Could you check a few things on this model? Use its own coordinates, in mm. Give positions to 0.01 mm unless a question says otherwise; leave off trailing zeros. Order: outer loops, then holes, each group sorted by start corner. A loop starts at its lowest first (then second) coordinate and runs counter-clockwise, first axis right, second up. Notation, with made-up numbers: M 8.5,74 L 50.5,74 A6 ccw 50.5,79 Z; hole C 43.5,64.5 d7. An arc over 180 degrees is marked long. Use a Markdown table: item, result. Add a question column.
Item 1: Suppose I cut it at B-B on z = 164. Write out the boundary of the cut face in (x, y) (3 decimals), plus the area to 3 significant figures.
Item 2: I'm going to push flat-ended pins straight in: pin 1 Ø3 at (x, z) = (1, -208) entering from +Y; pin 2 Ø5.5 at (x, z) = (0, -30) entering from +Y; pin 3 Ø0.6 at (y, z) = (8.5, 53) entering from +X. Where does each tip first touch, or does it pass through?
Item 3: Suppose I cut it at A-A on y = 3.5. Count the separate pieces of the cut face and the enclosed holes in it, plus the area to 3 significant figures.
Item 4: If I drill on L1, parallel to X at y = 1.35, z = 30; L2, parallel to X at y = 7, z = -150; L3, parallel to Y at x = -8.5, z = 46, over which ranges is the centre line in solid material (lowest first)? Write a range as from..to.
from build123d import *

# Parameters (mm, degrees)
BOSS_EXTRUDE1_DEPTH      = 230
BOSS_EXTRUDE1_DEPTH_BACK = 230


with BuildPart() as part:
    # Sketch1 → Boss-Extrude1 (new, two sides: drawn at the far end of the back side and taken through both)
    with BuildSketch(Plane.XY.offset(-BOSS_EXTRUDE1_DEPTH_BACK)):
        with BuildLine():
            Line((-10, 6.77615), (-10, 0.5))
            Line((-10, 0.5), (-9.5, 0))
            Line((-9.5, 0), (9.5, 0))
            Line((9.5, 0), (10, 0.5))
            Line((10, 0.5), (10, 6.77615))
            Line((10, 6.77615), (9.440021531, 7.099443113))
            ThreePointArc((9.440021531, 7.099443113), (9.015681976, 7.442706235), (8.71772889, 7.9))
            Line((8.71772889, 7.9), (7.5, 7.9))
            Line((7.5, 7.9), (7.5, 9.1))
            Line((7.5, 9.1), (8.71772889, 9.1))
            ThreePointArc((8.71772889, 9.1), (9.015681976, 9.557293765), (9.440021531, 9.900556887))
            Line((9.440021531, 9.900556887), (10, 10.22385))
            Line((10, 10.22385), (10, 10.7))
            Line((10, 10.7), (9.7, 11))
            Line((9.7, 11), (-9.7, 11))
            Line((-9.7, 11), (-10, 10.7))
            Line((-10, 10.7), (-10, 10.22385))
            Line((-10, 10.22385), (-9.440021531, 9.900556887))
            ThreePointArc((-9.440021531, 9.900556887), (-9.015681976, 9.557293765), (-8.71772889, 9.1))
            Line((-8.71772889, 9.1), (-7.5, 9.1))
            Line((-7.5, 9.1), (-7.5, 7.9))
            Line((-7.5, 7.9), (-8.71772889, 7.9))
            ThreePointArc((-8.71772889, 7.9), (-9.015681976, 7.442706235), (-9.440021531, 7.099443113))
            Line((-9.440021531, 7.099443113), (-10, 6.77615))
        make_face()
    extrude(amount=BOSS_EXTRUDE1_DEPTH + BOSS_EXTRUDE1_DEPTH_BACK)

    # Sketch2 → Cut-Revolve1 (revolve, cut)
    with BuildSketch(Plane(origin=(0, 0, 0), x_dir=(0, 0, -1), z_dir=(1, 0, 0)), mode=Mode.PRIVATE) as cut_revolve1_sk:
        Polygon((210, 11), (214.75, 11), (214.75, 5.5), (213, 5.5), (213, 0), (210, 0), align=None)
    revolve(cut_revolve1_sk.sketch.rotate(Axis((0, 0, -210), (0, 1, 0)), 180), axis=Axis((0, 0, -210), (0, 1, 0)), mode=Mode.SUBTRACT)

    # Sketch3 → Cut-Revolve2 (revolve, cut)
    with BuildSketch(Plane(origin=(0, 0, 0), x_dir=(0, 0, -1), z_dir=(1, 0, 0)), mode=Mode.PRIVATE) as cut_revolve2_sk:
        Polygon((150, 11), (154.75, 11), (154.75, 5.5), (153, 5.5), (153, 0), (150, 0), align=None)
    revolve(cut_revolve2_sk.sketch.rotate(Axis((0, 0, -150), (0, 1, 0)), 180), axis=Axis((0, 0, -150), (0, 1, 0)), mode=Mode.SUBTRACT)

    # Sketch4 → Cut-Revolve3 (revolve, cut)
    with BuildSketch(Plane(origin=(0, 0, 0), x_dir=(0, 0, -1), z_dir=(1, 0, 0)), mode=Mode.PRIVATE) as cut_revolve3_sk:
        Polygon((90, 11), (94.75, 11), (94.75, 5.5), (93, 5.5), (93, 0), (90, 0), align=None)
    revolve(cut_revolve3_sk.sketch.rotate(Axis((0, 0, -90), (0, 1, 0)), 180), axis=Axis((0, 0, -90), (0, 1, 0)), mode=Mode.SUBTRACT)

    # Sketch5 → Cut-Revolve4 (revolve, cut)
    with BuildSketch(Plane(origin=(0, 0, 0), x_dir=(0, 0, -1), z_dir=(1, 0, 0)), mode=Mode.PRIVATE) as cut_revolve4_sk:
        Polygon((30, 11), (34.75, 11), (34.75, 5.5), (33, 5.5), (33, 0), (30, 0), align=None)
    revolve(cut_revolve4_sk.sketch.rotate(Axis((0, 0, -30), (0, 1, 0)), 180), axis=Axis((0, 0, -30), (0, 1, 0)), mode=Mode.SUBTRACT)

    # Sketch6 → Cut-Revolve5 (revolve, cut)
    with BuildSketch(Plane(origin=(0, 0, 0), x_dir=(0, 0, -1), z_dir=(1, 0, 0)), mode=Mode.PRIVATE) as cut_revolve5_sk:
        Polygon((-30, 11), (-25.25, 11), (-25.25, 5.5), (-27, 5.5), (-27, 0), (-30, 0), align=None)
    revolve(cut_revolve5_sk.sketch.rotate(Axis((0, 0, 30), (0, 1, 0)), 180), axis=Axis((0, 0, 30), (0, 1, 0)), mode=Mode.SUBTRACT)

    # Sketch7 → Cut-Revolve6 (revolve, cut)
    with BuildSketch(Plane(origin=(0, 0, 0), x_dir=(0, 0, -1), z_dir=(1, 0, 0)), mode=Mode.PRIVATE) as cut_revolve6_sk:
        Polygon((-90, 11), (-85.25, 11), (-85.25, 5.5), (-87, 5.5), (-87, 0), (-90, 0), align=None)
    revolve(cut_revolve6_sk.sketch.rotate(Axis((0, 0, 90), (0, 1, 0)), 180), axis=Axis((0, 0, 90), (0, 1, 0)), mode=Mode.SUBTRACT)

    # Sketch8 → Cut-Revolve7 (revolve, cut)
    with BuildSketch(Plane(origin=(0, 0, 0), x_dir=(0, 0, -1), z_dir=(1, 0, 0)), mode=Mode.PRIVATE) as cut_revolve7_sk:
        Polygon((-150, 11), (-145.25, 11), (-145.25, 5.5), (-147, 5.5), (-147, 0), (-150, 0), align=None)
    revolve(cut_revolve7_sk.sketch.rotate(Axis((0, 0, 150), (0, 1, 0)), 180), axis=Axis((0, 0, 150), (0, 1, 0)), mode=Mode.SUBTRACT)

    # Sketch9 → Cut-Revolve8 (revolve, cut)
    with BuildSketch(Plane(origin=(0, 0, 0), x_dir=(0, 0, -1), z_dir=(1, 0, 0)), mode=Mode.PRIVATE) as cut_revolve8_sk:
        Polygon((-210, 11), (-205.25, 11), (-205.25, 5.5), (-207, 5.5), (-207, 0), (-210, 0), align=None)
    revolve(cut_revolve8_sk.sketch.rotate(Axis((0, 0, 210), (0, 1, 0)), 180), axis=Axis((0, 0, 210), (0, 1, 0)), mode=Mode.SUBTRACT)


solid = part.part
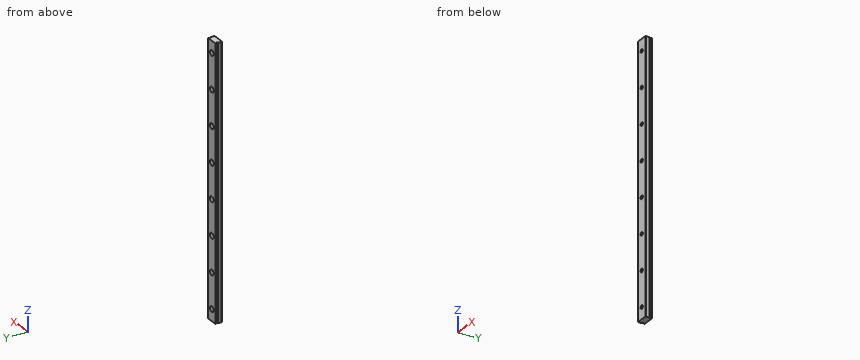
Findings below:
| question | item | result |
|---|---|---|
| 1 | outline | M -10,0.5 L -9.5,0 L 9.5,0 L 10,0.5 L 10,6.776 L 9.44,7.099 A1.75 cw 8.718,7.9 L 7.5,7.9 L 7.5,9.1 L 8.718,9.1 A1.75 cw 9.44,9.901 L 10,10.224 L 10,10.7 L 9.7,11 L -9.7,11 L -10,10.7 L -10,10.224 L -9.44,9.901 A1.75 cw -8.718,9.1 L -7.5,9.1 L -7.5,7.9 L -8.718,7.9 A1.75 cw -9.44,7.099 L -10,6.776 Z |
| 1 | area | 210 mm^2 |
| 2 | pin 1 | stops at y = 5.5 |
| 2 | pin 2 | passes through |
| 2 | pin 3 | stops at x = 7.5 |
| 3 | separate pieces | 1 |
| 3 | enclosed holes | 8 |
| 3 | area | 8,970 mm^2 |
| 4 | L1 | x = -10..-3, 3..10 |
| 4 | L2 | x = -9.61..-4.75, 4.75..9.61 |
| 4 | L3 | y = 0..7.9, 9.1..11 |
